```python
from build123d import *

# Parameters (mm, degrees)
F0_W     = 450
F0_H     = 450
F1_DEPTH = 950
F2_W     = 53.5874837637
F2_H     = 50
F2_H_2   = 450
F2_W_2   = 326.4125162363
F3_DEPTH = 450.001
F4_W     = 380
F4_H     = 425
F5_DEPTH = 450.001
F6_W     = 380
F6_H     = 233.320171364
F6_H_2   = 62.848264869
F7_DEPTH = 147.0908754191


with BuildPart() as f1:
    # F0 (on Top) → F1 (new body)
    with BuildSketch(Plane.XY):
        Rectangle(F0_W, F0_H)
    extrude(amount=F1_DEPTH)

    # F2 (on face) → F3 (cut, through all)
    with BuildSketch(Plane.YZ.offset(225)):
        Polygon((-225, 950), (-225, 500), (136.4125162363, 500), (190, 950), align=None)
        Polygon((225, 950), (171.4125162363, 500), (225, 500), align=None)
        with Locations((198.2062581182, 475)):
            Rectangle(F2_W, F2_H)
        with Locations((198.2062581182, 225)):
            Rectangle(F2_W, F2_H_2)
        with Locations((-26.7937418818, 225)):
            Rectangle(F2_W_2, F2_H_2)
    extrude(amount=-F3_DEPTH, mode=Mode.SUBTRACT)

    # F4 (on face) → F5 (cut, through all)
    with BuildSketch(Plane.XZ.offset(225)):
        with Locations((0, 212.5)):
            Rectangle(F4_W, F4_H)
    extrude(amount=-F5_DEPTH, mode=Mode.SUBTRACT)

    # F6 (on face) → F7 (cut, through all)
    with BuildSketch(Plane(origin=(0, 75.7960170498, -9.0260396289), x_dir=(1, 0, 0), z_dir=(0, -0.9929841149, 0.1182478225))):
        with Locations((0, 629.2826261481)):
            Rectangle(F6_W, F6_H)
        with Locations((0, 863.5165368001)):
            Rectangle(F6_W, F6_H_2)
    extrude(amount=-F7_DEPTH, mode=Mode.SUBTRACT)


solid = f1.part
```
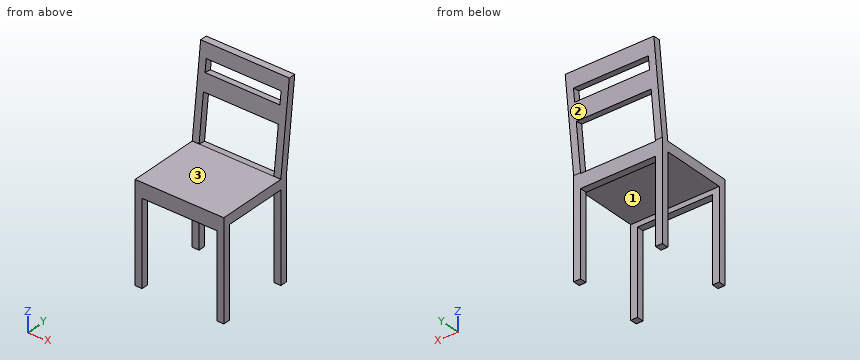
Verification items for the finished model (mm, model axes). Face numbers are marked on the shaded views. Give positions to 0.01 mm unless a question says otherwise; leave off trailing zeros. Loops run counter-clockwise (first coordinate to the right, second up) from the corner with the lowest first, then second, coordinate; pieces in that order, holes last.
1. Section check A-A, the plane z = 76. Enter the section's corners in (x, y), then the cut area to 3 significant figures.
2. Section check D-D, the plane y = -46. Enter the section's corners in (x, z).
3. Go/stop test with flat-tipped pins: pin 1 Ø17.5 at (x, y) = (2.5, -210) entering from -Z; pin 2 Ø1 at (x, y) = (-88, -139.5) entering from -Z. Record where each tip stops, or that it passes through.
4. Section check B-B, the plane x = -112. Enter the section's corners in (y, z), then the cut area to 3 significant figures.
5. Mould release check, pull along Y, two halves, no side actions. Record for the marked faces 1, 2 and 3: released by +Y, released by -Y, zero draft, split by the parting line, or undercut.
6. Thickness scan on line 1 (Z direction, x = 80.5, y = -143.5); line 2 (Y direction, x = 107.5, z = 757.5); line 3 (Y direction, x = -91, z = 887). Record the ranges inside material, lowest first.
7. Section check C-C, the plane z = 551. Enter the section's corners in (x, y).
Geometry says:
1. outline: (-225, -225) - (-190, -225) - (-190, -190) - (-225, -190) - close; (-225, 136.41) - (-190, 136.41) - (-190, 171.41) - (-225, 171.41) - close; (190, -225) - (225, -225) - (225, -190) - (190, -190) - close; (190, 136.41) - (225, 136.41) - (225, 171.41) - (190, 171.41) - close
1. area: 4,900 mm2
2. outline: (-225, 450) - (225, 450) - (225, 500) - (-225, 500) - close
3. pin 1: stops at z = 425
3. pin 2: stops at z = 450
4. outline: (-225, 425) - (-190, 425) - (-190, 450) - (136.41, 450) - (136.41, 425) - (171.41, 425) - (171.41, 495.83) - (136.41, 500) - (-225, 500) - close; (164, 731.68) - (198.51, 727.57) - (208.7, 813.12) - (174.19, 817.23) - close; (181.62, 879.64) - (216.13, 875.53) - (225, 950) - (190, 950) - close
4. area: 27,000 mm2
5. face 1: undercut
5. face 2: released by +Y
5. face 3: zero draft
6. line 1: z = 450 to 500
6. line 2: y = 167.08 to 202.08
6. line 3: y = 182.5 to 217.5
7. outline: (-225, 142.49) - (-190, 142.49) - (-190, 177.49) - (-225, 177.49) - close; (190, 142.49) - (225, 142.49) - (225, 177.49) - (190, 177.49) - close
